Source: CAD feature listing. Evaluate the final solid. Frame: model axes, mm. Face numbers are marked on the shaded views. A direction names the side the tool comes from. Coordinates: 2 decimals unless noted, no trailing zeros. Order: outer loops, then holes, each group sorted by start corner. A loop starts at its lowest first (then second) coordinate and runs counter-clockwise, first axis right, second up.
Item 1: Reachability of the marked faces 1, 2, 3, 4 and 5 from +Z, -Z, +X, -X, +Y, -Y: full face, straight path, thin tool, end or side. Return the list, or none.
Item 2: Contact query for flat-ended pins moving along their axis: P1, Ø1.5, axis at x = -23, z = -6.5, coming from the -Y side; P2, Ø0.6, axis at x = 1, y = 29, coming from the +Z side; P3, Ø8, axis at y = 4, z = 45.5, coming from the +X side. Output: stop coordinate, or through.
Item 3: Mould query, pull axis Y, two halves, no side actions, for the marked faces 6, 7 and 8. Classes: released by +Y, released by -Y, zero draft, split by the parting line, or undercut.
Item 4: Section D-D on y = 32.5. Return the cut outline in (x, z).
Item 5: Section C-C on z = 29.5. Return the cut outline in (x, y).
Item 6: Section A-A on z = 44.5. Return the cut outline in (x, y), then the cut area to 3 significant figures.
Item 7: Ray query, line 1 (Y direction, x = -30, z = 46); line 2 (Y direction, x = -7.5, z = 10); line 3 (Z direction, x = -24, y = 26). Return the intervals inside material, ascending.
from build123d import *

# Parameters (mm, degrees)
SKETCH1_W                = 50
SKETCH1_H                = 70
BOSS_EXTRUDE1_DEPTH      = 60
CUT_EXTRUDE1_DEPTH       = 60
SKETCH4_W                = 2.5
SKETCH4_H                = 2
SKETCH4_H_2              = 60
CUT_EXTRUDE2_DEPTH       = 95
SKETCH7_W                = 47.5
SKETCH7_H                = 45.554164346
CUT_EXTRUDE3_DEPTH       = 10
SKETCH8_R                = 2
BOSS_EXTRUDE2_DEPTH      = 2
BOSS_EXTRUDE2_DEPTH_BACK = 20
SKETCH9_W                = 6.754259693
SKETCH9_H                = 60
SKETCH9_W_2              = 7.009150451
SKETCH9_W_3              = 4.127603145
CUT_EXTRUDE4_DEPTH       = 2
SKETCH10_W               = 2
SKETCH10_H               = 4.127603145
SKETCH10_H_2             = 7.009150451
SKETCH10_H_3             = 6.754259693
CUT_EXTRUDE5_DEPTH       = 71
SKETCH11_R               = 0.75
CUT_EXTRUDE6_DEPTH       = 4


with BuildPart() as part:
    # Sketch1 → Boss-Extrude1 (new body)
    with BuildSketch(Plane(origin=(0, 0, 0), x_dir=(1, 0, 0), z_dir=(0, 1, 0))):
        with Locations((-20.864146805, -15.987939145)):
            Rectangle(SKETCH1_W, SKETCH1_H)
    extrude(amount=BOSS_EXTRUDE1_DEPTH)

    # Sketch2 → Cut-Extrude1 (cut)
    with BuildSketch(Plane(origin=(4.135853195, 0, 0), x_dir=(0, 0, -1), z_dir=(1, 0, 0))):
        Polygon((19.012060855, 50.122083557), (14.012060855, 55.122083557), (14.012060855, 4.877916443), (19.012060855, 9.877916443), align=None)
    extrude(amount=-CUT_EXTRUDE1_DEPTH, mode=Mode.SUBTRACT)

    # Sketch4 → Cut-Extrude2 (cut)
    with BuildSketch(Plane.XY.offset(50.987939145)):
        with Locations((-34.614146805, 59)):
            Rectangle(SKETCH4_W, SKETCH4_H)
        with Locations((-22.114146805, 59)):
            Rectangle(SKETCH4_W, SKETCH4_H)
        with Locations((-9.614146805, 59)):
            Rectangle(SKETCH4_W, SKETCH4_H)
        with Locations((2.885853195, 30)):
            Rectangle(SKETCH4_W, SKETCH4_H_2)
    extrude(amount=-CUT_EXTRUDE2_DEPTH, mode=Mode.SUBTRACT)

    # Sketch7 → Cut-Extrude3 (cut)
    with BuildSketch(Plane.XY.offset(50.987939145)):
        with Locations((-22.114146805, 22.777082173)):
            Rectangle(SKETCH7_W, SKETCH7_H)
    extrude(amount=-CUT_EXTRUDE3_DEPTH, mode=Mode.SUBTRACT)

    # Sketch8 → Boss-Extrude2 (add, two sides)
    with BuildSketch(Plane.XZ) as boss_extrude2_sk:
        with BuildLine():
            Line((-17.114146805, 40.987939145), (-27.114146805, 40.987939145))
            Line((-27.114146805, 40.987939145), (-27.114146805, 50.987939145))
            ThreePointArc((-27.114146805, 50.987939145), (-22.114146805, 55.987939145), (-17.114146805, 50.987939145))
            Line((-17.114146805, 50.987939145), (-17.114146805, 40.987939145))
        make_face()
        with Locations((-22.114146805, 50.987939145)):
            Circle(SKETCH8_R, mode=Mode.SUBTRACT)
    extrude(amount=BOSS_EXTRUDE2_DEPTH)
    extrude(boss_extrude2_sk.sketch, amount=-BOSS_EXTRUDE2_DEPTH_BACK)

    # Sketch9 → Cut-Extrude4 (cut)
    with BuildSketch(Plane(origin=(1.635853195, 0, 0), x_dir=(0, 0, -1), z_dir=(1, 0, 0))):
        with Locations((-27.243460969, 30)):
            Rectangle(SKETCH9_W, SKETCH9_H)
        with Locations((-7.48336392, 30)):
            Rectangle(SKETCH9_W_2, SKETCH9_H)
        with Locations((7.716086886, 30)):
            Rectangle(SKETCH9_W_3, SKETCH9_H)
    extrude(amount=-CUT_EXTRUDE4_DEPTH, mode=Mode.SUBTRACT)

    # Sketch10 → Cut-Extrude5 (cut)
    with BuildSketch(Plane(origin=(0, 60, 0), x_dir=(1, 0, 0), z_dir=(0, 1, 0))):
        with Locations((-44.864146805, 7.716086886)):
            Rectangle(SKETCH10_W, SKETCH10_H)
        with Locations((-44.864146805, -7.48336392)):
            Rectangle(SKETCH10_W, SKETCH10_H_2)
        with Locations((-44.864146805, -27.243460969)):
            Rectangle(SKETCH10_W, SKETCH10_H_3)
    extrude(amount=-CUT_EXTRUDE5_DEPTH, mode=Mode.SUBTRACT)

    # Sketch11 → Cut-Extrude6 (cut)
    with BuildSketch(Plane(origin=(-17.114146805, 0, 0), x_dir=(0, 0, -1), z_dir=(1, 0, 0))):
        with Locations((-50.987939145, 15.146186294)):
            Circle(SKETCH11_R)
    extrude(amount=-CUT_EXTRUDE6_DEPTH, mode=Mode.SUBTRACT)


solid = part.part
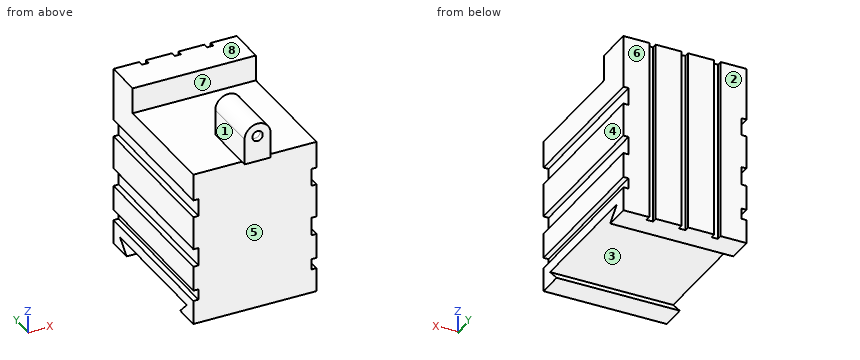
Answer list:
1. face 1: +Z, -X, -Y
1. face 2: +Z, -Z, +X, -X, +Y
1. face 3: +X, -X
1. face 4: +Z, -Z, +X, +Y, -Y
1. face 5: -Z, +X, -X, -Y
2. P1: stops at y = 0
2. P2: stops at z = 40.99
2. P3: stops at x = -17.11
3. face 6: released by +Y
3. face 7: undercut
3. face 8: zero draft
4. outline: (-45.86, -14.01) - (1.64, -14.01) - (1.64, -9.78) - (-0.36, -9.78) - (-0.36, -5.65) - (1.64, -5.65) - (1.64, 3.98) - (-0.36, 3.98) - (-0.36, 10.99) - (1.64, 10.99) - (1.64, 23.87) - (-0.36, 23.87) - (-0.36, 30.62) - (1.64, 30.62) - (1.64, 40.99) - (-45.86, 40.99) - (-45.86, 30.62) - (-43.86, 30.62) - (-43.86, 23.87) - (-45.86, 23.87) - (-45.86, 10.99) - (-43.86, 10.99) - (-43.86, 3.98) - (-45.86, 3.98) - (-45.86, -5.65) - (-43.86, -5.65) - (-43.86, -9.78) - (-45.86, -9.78) - close
5. outline: (-43.86, 0) - (-0.36, 0) - (-0.36, 60) - (-8.36, 60) - (-8.36, 58) - (-10.86, 58) - (-10.86, 60) - (-20.86, 60) - (-20.86, 58) - (-23.36, 58) - (-23.36, 60) - (-33.36, 60) - (-33.36, 58) - (-35.86, 58) - (-35.86, 60) - (-43.86, 60) - close
6. outline: (-45.86, 45.55) - (1.64, 45.55) - (1.64, 60) - (-8.36, 60) - (-8.36, 58) - (-10.86, 58) - (-10.86, 60) - (-20.86, 60) - (-20.86, 58) - (-23.36, 58) - (-23.36, 60) - (-33.36, 60) - (-33.36, 58) - (-35.86, 58) - (-35.86, 60) - (-45.86, 60) - close; (-27.11, -2) - (-17.11, -2) - (-17.11, 20) - (-27.11, 20) - close
6. area: 891 mm2
7. line 1: y = 45.55 to 60
7. line 2: y = 0 to 60
7. line 3: z = -14.01 to 40.99
